from build123d import *

# Parameters (mm, degrees)
BASPROSKE_W        = 12.7
BASPROSKE_H        = 20.6375
TOOTHCUT_DEPTH     = 32.829276029
TEETHCUTS_COUNT    = 24
TEETHCUTS_ANGLE    = 345
BORSKE_R           = 7.9375
BORE_DEPTH         = 50.8000508
KEYSKE_W           = 4.7625
KEYSKE_H           = 9.2837
KEYWAY_DEPTH       = 50.8000508
SKETCH2_W          = 4.7625
SKETCH2_H          = 0.7874
CUT_EXTRUDE2_DEPTH = 32.669469117


with BuildPart() as part:
    # BasProSke → Base-Revolve (revolve)
    with BuildSketch(Plane(origin=(0, 0, 0), x_dir=(1, 0, 0), z_dir=(0, 1, 0)), mode=Mode.PRIVATE) as base_revolve_sk:
        with Locations((6.35, 10.31875)):
            Rectangle(BASPROSKE_W, BASPROSKE_H)
    revolve(base_revolve_sk.sketch.rotate(Axis((-10, 0, 0), (1, 0, 0)), 180), axis=Axis((-10, 0, 0), (1, 0, 0)))

    # TooCutSke → ToothCut (cut, through all)
    with BuildSketch(Plane(origin=(0, 0, 0), x_dir=(0, 0, -1), z_dir=(1, 0, 0))):
        with BuildLine():
            ThreePointArc((0.762542858, 17.047308877), (0, 17.064355), (-0.762542858, 17.047308877))
            ThreePointArc((-0.762542858, 17.047308877), (-1.295412414, 18.888113288), (-2.270705673, 20.537753824))
            ThreePointArc((-2.270705673, 20.537753824), (0, 20.6629), (2.270705673, 20.537753824))
            ThreePointArc((2.270705673, 20.537753824), (1.295412414, 18.888113288), (0.762542858, 17.047308877))
        make_face()
    toothcut = extrude(amount=TOOTHCUT_DEPTH, mode=Mode.SUBTRACT)

    # TeethCuts: ToothCut ×24 about axis
    teethcuts_axis = Axis((-10, 0, 0), (1, 0, 0))
    for i in range(1, TEETHCUTS_COUNT):
        add(toothcut.rotate(teethcuts_axis, i * TEETHCUTS_ANGLE / (TEETHCUTS_COUNT - 1)), mode=Mode.SUBTRACT)

    # BorSke → Bore (cut, symmetric)
    with BuildSketch(Plane(origin=(0, 0, 0), x_dir=(0, 0, -1), z_dir=(1, 0, 0))):
        with Locations(Location((0, 0, 0), (0, 0, 180))):
            Circle(BORSKE_R)
    extrude(amount=BORE_DEPTH, both=True, mode=Mode.SUBTRACT)

    # KeySke → Keyway (cut, symmetric)
    with BuildSketch(Plane(origin=(0, 0, 0), x_dir=(0, 0, -1), z_dir=(1, 0, 0))):
        with Locations((0, 4.64185)):
            Rectangle(KEYSKE_W, KEYSKE_H)
    extrude(amount=KEYWAY_DEPTH, both=True, mode=Mode.SUBTRACT)

    # Sketch2 → Cut-Extrude2 (cut, through all)
    with BuildSketch(Plane(origin=(12.7, 0, 0), x_dir=(0, 0, -1), z_dir=(1, 0, 0))):
        with Locations((0, 9.6774)):
            Rectangle(SKETCH2_W, SKETCH2_H)
    extrude(amount=-CUT_EXTRUDE2_DEPTH, mode=Mode.SUBTRACT)


solid = part.part
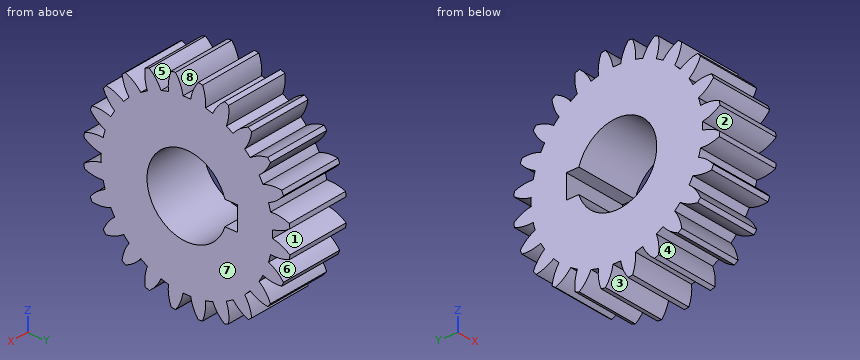
The listing builds one solid part. Answer for the finished solid, in the listing's coordinates (mm). Face numbers are marked on the shaded views. A direction names the side the tool comes from. Round coordinates to 2 decimals unless told otherwise and drop trailing zeros. Loops run counter-clockwise (first coordinate to the right, second up) from the corner with the lowest first, then second, coordinate; pieces in that order, holes last. Notation, with made-up numbers: M 86.25,57.25 L 142.25,57.25 A20 ccw 142.25,65.25 Z; hole C 3.5,3 d11. An arc over 180 degrees is marked long. Return JSON: item names as keys, results as strings.
Q1. The mould has two halves that part along Y. Classify the marked faces 6, 7 and 8: released by +Y, released by -Y, zero draft, split by the parting line, or undercut.
Results list:
{"face 6": "released by +Y", "face 7": "zero draft", "face 8": "undercut"}
Q2. Find section B-B, the plane z = -6.5. Determine the outline of the cut face in (x, y).
Results list:
{"outline": "M 0,-18.33 L 12.7,-18.33 L 12.7,-4.56 L 0,-4.56 Z; M 0,4.56 L 12.7,4.56 L 12.7,18.33 L 0,18.33 Z"}
Q3. Which of the six approach directions +Z, -Z, +X, -X, +Y, -Y give full straight-line access (tool end or side, diameter ignored) to the marked faces 1, 2, 3, 4 and 5?
Results list:
{"face 1": "+X, -X, +Y", "face 2": "+X, -X, -Y", "face 3": "-Z, +X, -X", "face 4": "+X, -X", "face 5": "+Z, +X, -X"}
Q4. Find the intervals of material crossed by line 1 along Z through (x, y) = (2.5, -17.5); line 2 along Z through (x, y) = (4.5, 0); line 3 along Y through (x, z) = (5, -12), in increasing order. Write a range as from..to.
Results list:
{"line 1": "z = -8.36..-5.84, -3.72..-0.85, 0.85..3.72, 5.84..8.36", "line 2": "z = -17.06..-7.94, 7.94..17.06", "line 3": "y = -16.55..-13.35, -12.13..12.13, 13.35..16.55"}
Q5. Each of these flat-tipped pins is pushed along its axis until it touches: pin 1 Ø1.5 at (x, y) = (2.5, -3.5) entering from +Z; pin 2 Ø2.5 at (x, y) = (9, 9) entering from +Z; pin 3 Ø2 at (x, y) = (3, 15) entering from -Z. Where does it stop, or does it pass through?
Results list:
{"pin 1": "stops at z = 20.45", "pin 2": "stops at z = 19.13", "pin 3": "stops at z = -12.9"}
Q6. Find section A-A, the plane y = 0. Determine the outline of the cut face in (x, z), plus the area to 3 significant figures.
Results list:
{"outline": "M 0,-17.06 L 12.7,-17.06 L 12.7,-7.94 L 0,-7.94 Z; M 0,7.94 L 12.7,7.94 L 12.7,17.06 L 0,17.06 Z", "area": "232 mm2"}
